Work out the finished part from the listing and answer in its coordinate system (mm). Face numbers are marked on the shaded views. A direction names the side the tool comes from. Coordinates: 2 decimals unless noted, no trailing zeros. Order: outer loops, then holes, each group sorted by start corner. A loop starts at its lowest first (then second) coordinate and runs counter-clockwise, first axis right, second up. Notation, with made-up numbers: (6, -34.5) -> (33, -34.5) arc R25 cw to (33, 4.5) -> close; hole circle Ø8 at (-1, 30). An arc over 180 degrees is marked (long way). Write item = value, one per line. Start each with the question number.
Q1. Flat-ended cylindrical pins translate along their axes: pin 1 (5 mm diameter, centred on x = 3, y = 48, fed in from +Z); pin 2 (8 mm diameter, centred on x = 26.5, y = 16.5, fed in from +Z); pin 3 (3 mm diameter, centred on x = 26, y = 3, fed in from -Z); pin 4 (4.5 mm diameter, centred on x = 8, z = 4, fed in from +Y). Find the tip coordinate at first contact, or state that the pin passes through.
Q2. For a pull along X with two mould halves and no side action, classify the marked faces 1, 2 and 3 as +X half, -X half, draft (parallel to the pull), parting line (faces both ways), or undercut.
Q3. Which of the six approach directions +Z, -Z, +X, -X, +Y, -Y give full straight-line access (tool end or side, diameter ignored) to the marked faces 4, 5, 6, 7 and 8?
Q4. The part is cut by section C-C, the plane x = 19. Determine the outline of the cut face in (y, z).
Q5. The part is cut by section A-A, the plane y = 7. Determine the outline of the cut face in (x, z), plus the area to 3 significant figures.
Q6. The part is cut by section B-B, the plane x = 13. Determine the outline of the cut face in (y, z), plus the area to 3 significant figures.
Q7. Straight lines are drawn through the part: L1, parallel to Y at x = 34, z = 4; L2, parallel to X at y = 50.5, z = 4; L3, parallel to Y at x = 13, z = 5. For each, find the intervals that lie inside material, in ascending order. Write a range as from..to.
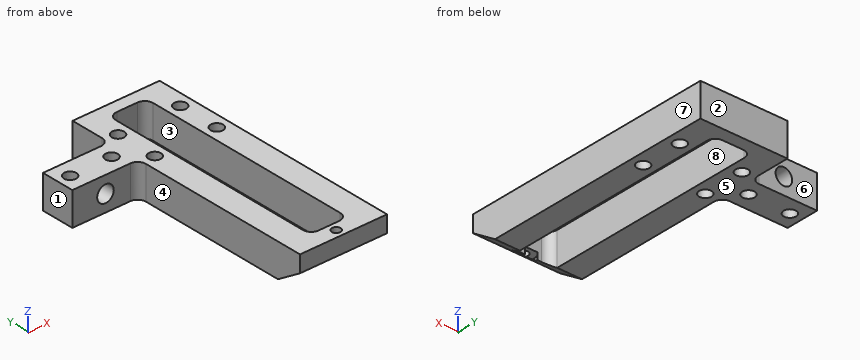
```python
from build123d import *

# Parameters (mm, degrees)
SKETCH_1_R          = 1.5
EXTRUDE_1_DEPTH     = 8
FILLET_1_R          = 2
SKETCH_2_W          = 9
SKETCH_2_H          = 55
CUT_EXTRUDE_1_DEPTH = 73.642962495
FILLET_2_R          = 2
SKETCH_3_R          = 2
CUT_EXTRUDE_2_DEPTH = 59.043087444
SKETCH_4_R          = 1.05
CUT_EXTRUDE_3_DEPTH = 73.642962495
SKETCH_5_R          = 2.5
CUT_EXTRUDE_4_DEPTH = 3
CUT_EXTRUDE_5_DEPTH = 22


with BuildPart() as part:
    # 草图1 → 凸台-拉伸1 (new body)
    with BuildSketch(Plane.XY):
        Polygon((37, 62), (37, 0), (16, 0), (16, 44), (0, 44), (0, 52), (16, 52), (16, 62), align=None)
        with Locations((19, 53)):
            Circle(SKETCH_1_R, mode=Mode.SUBTRACT)
        with Locations((34, 53)):
            Circle(SKETCH_1_R, mode=Mode.SUBTRACT)
        with Locations((19, 43)):
            Circle(SKETCH_1_R, mode=Mode.SUBTRACT)
        with Locations((34, 43)):
            Circle(SKETCH_1_R, mode=Mode.SUBTRACT)
        with Locations((3, 48)):
            Circle(SKETCH_1_R, mode=Mode.SUBTRACT)
        with Locations((13, 48)):
            Circle(SKETCH_1_R, mode=Mode.SUBTRACT)
    extrude(amount=EXTRUDE_1_DEPTH)

    # 圆角1
    fillet_1_edges = [part.edges().sort_by_distance(p)[0] for p in [
        (16, 52, 4),
        (16, 44, 4),
    ]]
    fillet(fillet_1_edges, radius=FILLET_1_R)

    # 草图2 → 切除-拉伸1 (cut, through all)
    with BuildSketch(Plane.XY.offset(8)):
        with Locations((26.5, 31.5)):
            Rectangle(SKETCH_2_W, SKETCH_2_H)
    extrude(amount=-CUT_EXTRUDE_1_DEPTH, mode=Mode.SUBTRACT)

    # 圆角2
    fillet_2_edges = [part.edges().sort_by_distance(p)[0] for p in [
        (31, 59, 4),
        (31, 4, 4),
        (22, 4, 4),
        (22, 59, 4),
    ]]
    fillet(fillet_2_edges, radius=FILLET_2_R)

    # 草图3 → 切除-拉伸2 (cut, through all)
    with BuildSketch(Plane.XZ.offset(-44)):
        with Locations(Location((8, 4, 0), (0, 0, 270))):
            Circle(SKETCH_3_R)
    extrude(amount=-CUT_EXTRUDE_2_DEPTH, mode=Mode.SUBTRACT)

    # 草图4 → 切除-拉伸3 (cut, through all)
    with BuildSketch(Plane.XY.offset(8)):
        with Locations((26.5, 2)):
            Circle(SKETCH_4_R)
    extrude(amount=-CUT_EXTRUDE_3_DEPTH, mode=Mode.SUBTRACT)

    # 草图5 → 切除-拉伸4 (cut)
    with BuildSketch(Plane(origin=(0, 0, 0), x_dir=(-1, 0, 0), z_dir=(0, 0, -1))):
        with Locations((-26.5, 2)):
            Circle(SKETCH_5_R)
    extrude(amount=-CUT_EXTRUDE_4_DEPTH, mode=Mode.SUBTRACT)

    # 草图6 → 切除-拉伸5 (cut)
    with BuildSketch(Plane(origin=(37, 0, 0), x_dir=(0, 0, -1), z_dir=(1, 0, 0))):
        Polygon((-4, 0), (0, 6), (0, 0), align=None)
    extrude(amount=-CUT_EXTRUDE_5_DEPTH, mode=Mode.SUBTRACT)


solid = part.part
```
Model answer:
q1.pin_1 = 8
q1.pin_2 = through
q1.pin_3 = 1.33
q1.pin_4 = 52
q2.face_1 = -X half
q2.face_2 = draft
q2.face_3 = undercut
q3.face_4 = +Z, -Z, -X, -Y
q3.face_5 = -Z, +X, -X, +Y, -Y
q3.face_6 = +Z, -Z, -X, +Y
q3.face_7 = +Z, -Z, +X, +Y, -Y
q3.face_8 = +Z, -Z
q4.outline = (0, 4) -> (6, 0) -> (41.5, 0) -> (41.5, 8) -> (0, 8) -> close; (44.5, 0) -> (51.5, 0) -> (51.5, 8) -> (44.5, 8) -> close; (54.5, 0) -> (62, 0) -> (62, 8) -> (54.5, 8) -> close
q5.outline = (16, 0) -> (22, 0) -> (22, 8) -> (16, 8) -> close; (31, 0) -> (37, 0) -> (37, 8) -> (31, 8) -> close
q5.area = 96.0 mm2
q6.outline = (44, 0) -> (46.5, 0) -> (46.5, 8) -> (44, 8) -> close; (49.5, 0) -> (52, 0) -> (52, 8) -> (49.5, 8) -> close
q6.area = 40.0 mm2
q7.L1 = 0..41.5, 44.5..51.5, 54.5..62
q7.L2 = 0..6, 10..22, 31..37
q7.L3 = 44..46.5, 49.5..52
